Design review of the part built by this model. Coordinates are the model's own, in mm. A direction names the side the tool comes from. Coordinates: 2 decimals unless noted, no trailing zeros. Order: outer loops, then holes, each group sorted by start corner. A loop starts at its lowest first (then second) coordinate and runs counter-clockwise, first axis right, second up. Notation, with made-up numbers: (29.25, -20) -> (61.25, -20) arc R19 ccw to (61.25, 5) -> close; hole circle Ø2 at (36, 60). An arc over 180 degrees is marked (long way). Write item = value, one per line.
```python
from build123d import *

# Parameters (mm, degrees)
F1_DEPTH = 10


with BuildPart() as f1:
    # F0 (on Top) → F1 (new body)
    with BuildSketch(Plane.XY):
        with BuildLine():
            Line((-4.861253, -2), (-1, -2))
            Line((-1, -2), (-1, 1))
            ThreePointArc((-1, 1), (-1.292893, 1.707107), (-2, 2))
            Line((-2, 2), (-6.726452, 2))
            ThreePointArc((-6.726452, 2), (-6.91988, 1.91988), (-7, 1.726452))
            Line((-7, 1.726452), (-7, -1.726452))
            ThreePointArc((-7, -1.726452), (-6.91988, -1.91988), (-6.726452, -2))
            Line((-6.726452, -2), (-4.861253, -2))
        make_face()
        with BuildLine():
            Line((1, -2), (4.861253, -2))
            Line((4.861253, -2), (6.726452, -2))
            ThreePointArc((6.726452, -2), (6.91988, -1.91988), (7, -1.726452))
            Line((7, -1.726452), (7, 1.726452))
            ThreePointArc((7, 1.726452), (6.91988, 1.91988), (6.726452, 2))
            Line((6.726452, 2), (2, 2))
            ThreePointArc((2, 2), (1.292893, 1.707107), (1, 1))
            Line((1, 1), (1, -2))
        make_face()
        Polygon((0.5, -2.699547), (0.5, -6.570132), (4.861253, -6.570132), (4.861253, -2), (1, -2), (1, -2.699547), align=None)
        Polygon((-1, -2.699547), (-1, -2), (-4.861253, -2), (-4.861253, -6.570132), (-0.5, -6.570132), (-0.5, -2.699547), align=None)
        with BuildLine():
            Line((-0.5, -1.483021), (-0.5, -2.699547))
            Line((-0.5, -2.699547), (-0.5, -6.570132))
            Line((-0.5, -6.570132), (0, -6.570132))
            Line((0, -6.570132), (0.5, -6.570132))
            Line((0.5, -6.570132), (0.5, -2.699547))
            Line((0.5, -2.699547), (0.5, -1.483021))
            ThreePointArc((0.5, -1.483021), (0, -1.983021), (-0.5, -1.483021))
        make_face()
        with BuildLine():
            ThreePointArc((0.5, -1.483021), (0, -0.983021), (-0.5, -1.483021))
            Line((-0.5, -1.483021), (0.5, -1.483021))
        make_face()
        with BuildLine():
            Line((0.5, -1.483021), (-0.5, -1.483021))
            ThreePointArc((-0.5, -1.483021), (0, -1.983021), (0.5, -1.483021))
        make_face()
    extrude(amount=F1_DEPTH)


solid = f1.part
```
(1) We need section A-A (y = 0.5). Write out the cut boundary in (x, z), and give its area (3 significant figures).
Report:
outline = (-7, 0) -> (-1, 0) -> (-1, 10) -> (-7, 10) -> close; (1, 0) -> (7, 0) -> (7, 10) -> (1, 10) -> close
area = 120 mm²
(2) Insertion check: pin 1 (0.6 mm diameter, centred on x = 0.5, z = 6, fed in from +Y); pin 2 (0.6 mm diameter, centred on x = -5.5, z = 3.5, fed in from -Y); pin 3 (1.4 mm diameter, centred on y = -4.5, z = 4.5, fed in from +X). Each pin has a flat end and moves straight along its axis. Give the tip position at first contact, or say it passes through.
Report:
pin_1 = -1.02
pin_2 = -2
pin_3 = 4.86
(3) The part is to be moulded in two halves that separate along X. For faces 4 (the flat face through (0, -2, 0)), 5 (the flat face through (-7, 0, 5)), 6 (the flat face through (-1, -1, 5)), say which applies: released by +X, released by -X, zero draft, split by the parting line, or undercut.
Report:
face_4 = zero draft
face_5 = released by -X
face_6 = undercut
(4) We need section B-B (z = 6.25). Write out the cut boundary in (x, y), and give its area (4 significant figures).
Report:
outline = (-7, -1.73) arc R0.27 ccw to (-6.73, -2) -> (-4.86, -2) -> (-4.86, -6.57) -> (4.86, -6.57) -> (4.86, -2) -> (6.73, -2) arc R0.27 ccw to (7, -1.73) -> (7, 1.73) arc R0.27 ccw to (6.73, 2) -> (2, 2) arc R1 ccw to (1, 1) -> (1, -2.7) -> (0.5, -2.7) -> (0.5, -1.48) arc R0.5 ccw to (-0.5, -1.48) -> (-0.5, -2.7) -> (-1, -2.7) -> (-1, 1) arc R1 ccw to (-2, 2) -> (-6.73, 2) arc R0.27 ccw to (-7, 1.73) -> close
area = 92.15 mm²
(5) We need section C-C (y = -1.25). Write out the cut boundary in (x, z).
Report:
outline = (-7, 0) -> (-1, 0) -> (-1, 10) -> (-7, 10) -> close; (-0.44, 0) -> (0.44, 0) -> (0.44, 10) -> (-0.44, 10) -> close; (1, 0) -> (7, 0) -> (7, 10) -> (1, 10) -> close
(6) For L1, parallel to X at y = -2.5, z = 5.5; L2, parallel to X at y = -1.25, z = 4.75; L3, parallel to X at y = 1, z = 6, list the stretches that pass through material, from the lowest coordinate up.
Report:
L1 = -4.86 to -1, -0.5 to 0.5, 1 to 4.86
L2 = -7 to -1, -0.44 to 0.44, 1 to 7
L3 = -7 to -1, 1 to 7
(7) We need section D-D (x = 0.25). Write out the cut boundary in (y, z).
Report:
outline = (-6.57, 0) -> (-1.05, 0) -> (-1.05, 10) -> (-6.57, 10) -> close
(8) For faces 1 (the flat face through (6, -2, 5)), 2 (the flat face through (-6, -2, 5)), 3 (the flat face through (-0.5, -2, 5)), list the 3-axis set-ups (+Z, -Z, +X, -X, +Y, -Y) from which the entire face can be reached by the end or side of a thin tool; tool diameter is ignored.
Report:
face_1 = +Z, -Z, +X, -Y
face_2 = +Z, -Z, -X, -Y
face_3 = +Z, -Z, +Y
